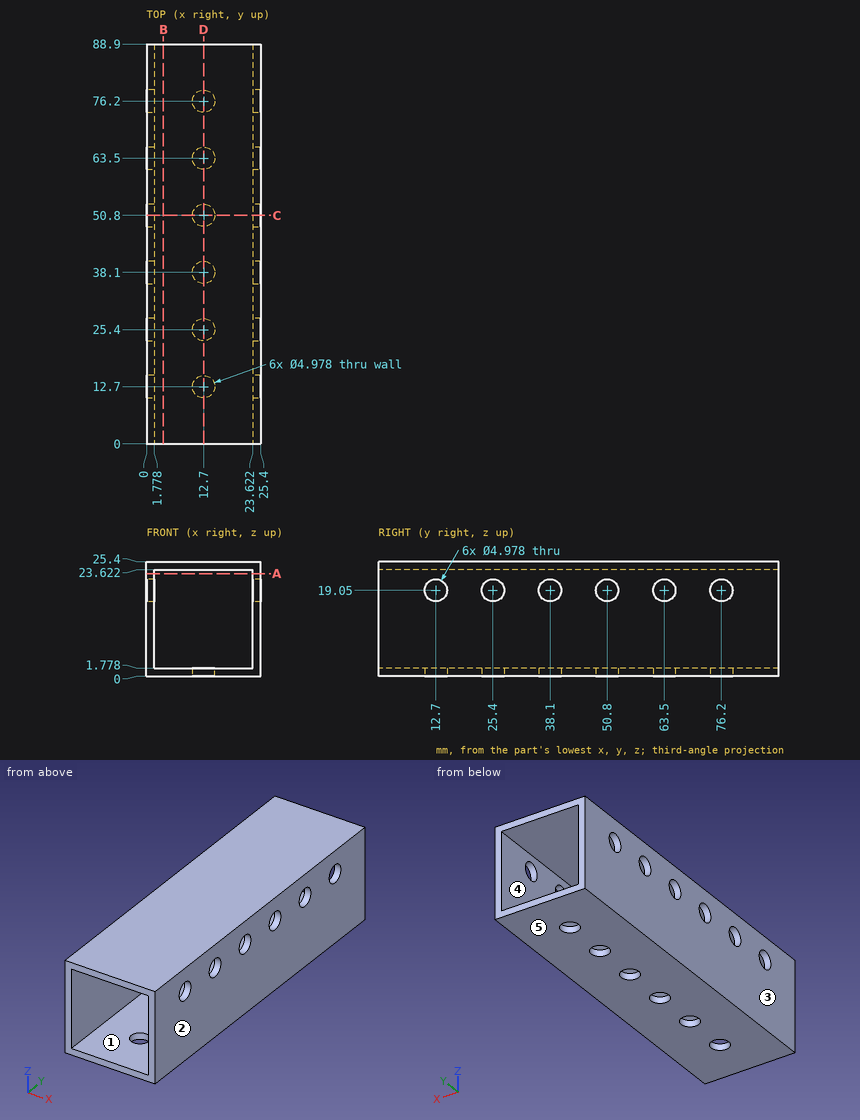
Print and shaded views of the part. All mm, measured from the part's lowest x, y and z. A direction names the side the tool comes from. Coordinates: 2 decimals unless noted, no trailing zeros. Write each loop counter-clockwise with the first axis right and the second up, starting at its lowest first coordinate (ties: lowest second). Pieces come first, ordered by that corner, then holes. Notation, with made-up numbers: M 47.25,21 L 54.25,21 A7 cw 54.25,28 Z; hole C 59.5,26.25 d11. An arc over 180 degrees is marked long. Return JSON: item names as keys, results as strings.
1. Saw through at D-D, the plane x = 12.7. Count the separate pieces of the cut face and the enclosed holes in it, then the cut area to 3 significant figures.
Determined:
{"separate pieces": "8", "enclosed holes": "0", "area": "263 mm²"}
2. Pull direction X, two halves, no side cores. Call the marked faces 3, 4 and 5: pulls with the +X half, pulls with the -X half, needs draft (parallel to the pull), parting line crosses it, or undercut.
Determined:
{"face 3": "pulls with the -X half", "face 4": "undercut", "face 5": "needs draft"}
3. 3-axis set-ups, long thin cutter, end or side, ignore diameter. For the marked faces 1 and 2: which of +Z, -Z, +X, -X, +Y, -Y reach the whole face in a straight line?
Determined:
{"face 1": "+Y, -Y", "face 2": "+Z, -Z, +X, +Y, -Y"}
4. Saw through at C-C, the plane y = 50.8. Write the cut outline in (x, z).
Determined:
{"outline": "M 0,0 L 10.21,0 L 10.21,1.78 L 1.78,1.78 L 1.78,16.56 L 0,16.56 Z; M 0,21.54 L 1.78,21.54 L 1.78,23.62 L 23.62,23.62 L 23.62,21.54 L 25.4,21.54 L 25.4,25.4 L 0,25.4 Z; M 15.19,0 L 25.4,0 L 25.4,16.56 L 23.62,16.56 L 23.62,1.78 L 15.19,1.78 Z"}
5. Saw through at A-A, the plane z = 22.75. Write the cut outline in (x, y), then the cut area to 3 significant figures.
Determined:
{"outline": "M 0,0 L 1.78,0 L 1.78,88.9 L 0,88.9 Z; M 23.62,0 L 25.4,0 L 25.4,88.9 L 23.62,88.9 Z", "area": "316 mm²"}
6. Flat gauge pins, fed straight in: pin 1 Ø3 at (x, y) = (12.7, 76.2) entering from -Z; pin 2 Ø4.5 at (y, z) = (63.5, 19.05) entering from +X. Where does each tip first touch, or does it go through?
Determined:
{"pin 1": "z = 23.62", "pin 2": "through"}
7. Probe L1, parallel to X at y = 56, z = 9; L2, parallel to Z at x = 24.95, y = 63.5. List the from-to ranges inside material, lowest first.
Determined:
{"L1": "0 to 1.78, 23.62 to 25.4", "L2": "0 to 16.56, 21.54 to 25.4"}
8. Saw through at B-B, the plane x = 3.75. Write the cut outline in (y, z), then the cut area to 3 significant figures.
Determined:
{"outline": "M 0,0 L 88.9,0 L 88.9,1.78 L 0,1.78 Z; M 0,23.62 L 88.9,23.62 L 88.9,25.4 L 0,25.4 Z", "area": "316 mm²"}
